Build history of the part. All positions in model axes, mm. Face numbers are marked on the shaded views. A direction names the side the tool comes from. Coordinates: 2 decimals unless noted, no trailing zeros.
from build123d import *
from OCP.BRepFilletAPI import BRepFilletAPI_MakeChamfer

# Parameters (mm, degrees)
SKETCH1_W                       = 194
SKETCH1_H                       = 90
BOSS_EXTRUDE1_DEPTH             = 7
SKETCH3_W                       = 194
SKETCH3_H                       = 90
SKETCH2_W                       = 150
SKETCH2_H                       = 70
CHAMFER1_SIZE                   = 2
SKETCH4_R                       = 2.15
CUT_EXTRUDE1_DEPTH              = 7
SKETCH5_W                       = 150
SKETCH5_H                       = 60
CUT_EXTRUDE2_DEPTH              = 36
SKETCH6_W                       = 150
SKETCH6_H                       = 64
CUT_EXTRUDE3_DEPTH              = 32
SKETCH7_W                       = 6
SKETCH7_H                       = 64
CUT_EXTRUDE4_DEPTH              = 4
SKETCH8_R                       = 2.05
CUT_EXTRUDE5_DEPTH              = 6
CHAMFER2_SIZE                   = 1
CHAMFER2_SIZE2                  = 0.615681714
CHAMFER2_SIZE2_2                = 0.436631997
CHAMFER3_SIZE                   = 0.6
SKIZZE1_W                       = 54.050484576
SKIZZE1_H                       = 12.5
SKIZZE1_W_2                     = 40
SKIZZE1_H_2                     = 21.453027382
AUFSATZ_LINEAR_AUSTRAGEN1_DEPTH = 10
SKIZZE3_W                       = 47.974757712
SKIZZE3_H                       = 1
SCHNITT_LINEAR_AUSTRAGEN2_DEPTH = 4
SKETCH9_W                       = 150
SKETCH9_H                       = 64
CUT_EXTRUDE6_DEPTH              = 32
CHAMFER4_SIZE                   = 0.4


with BuildPart() as part:
    # Sketch1 → Boss-Extrude1 (new body)
    with BuildSketch(Plane(origin=(0, 0, 0), x_dir=(1, 0, 0), z_dir=(0, 1, 0))):
        Rectangle(SKETCH1_W, SKETCH1_H)
    extrude(amount=BOSS_EXTRUDE1_DEPTH)

    # Sketch3 → Loft2 section 0
    with BuildSketch(Plane(origin=(0, 7, 0), x_dir=(1, 0, 0), z_dir=(0, 1, 0))):
        Rectangle(SKETCH3_W, SKETCH3_H)
    # Sketch2 → Loft2 section 1
    with BuildSketch(Plane(origin=(0, 37, 0), x_dir=(1, 0, 0), z_dir=(0, 1, 0))):
        Rectangle(SKETCH2_W, SKETCH2_H)
    loft()

    # Chamfer1
    chamfer1_edges = [part.edges().sort_by_distance(p)[0] for p in [
        (-97, 3.5, 45),
        (97, 3.5, 45),
        (97, 3.5, -45),
        (-97, 3.5, -45),
    ]]
    chamfer(chamfer1_edges, length=CHAMFER1_SIZE)

    # Sketch4 → Cut-Extrude1 (cut)
    with BuildSketch(Plane.XZ):
        with Locations(Location((40, -41.5, 0), (0, 0, 270))):
            Circle(SKETCH4_R)
        with Locations(Location((-40, -41.5, 0), (0, 0, 270))):
            Circle(SKETCH4_R)
    cut_extrude1 = extrude(amount=-CUT_EXTRUDE1_DEPTH, mode=Mode.SUBTRACT)

    # Sketch5 → Cut-Extrude2 (cut)
    with BuildSketch(Plane.XZ):
        Rectangle(SKETCH5_W, SKETCH5_H)
    extrude(amount=-CUT_EXTRUDE2_DEPTH, mode=Mode.SUBTRACT)

    # Mirror1: Cut-Extrude1 across plane
    add(cut_extrude1.mirror(Plane.XY), mode=Mode.SUBTRACT)

    # Sketch6 → Cut-Extrude3 (cut)
    with BuildSketch(Plane.XZ):
        Rectangle(SKETCH6_W, SKETCH6_H)
    extrude(amount=-CUT_EXTRUDE3_DEPTH, mode=Mode.SUBTRACT)

    # Sketch7 → Cut-Extrude4 (cut)
    with BuildSketch(Plane.XZ):
        with Locations((-78, 0)):
            Rectangle(SKETCH7_W, SKETCH7_H)
        with Locations((78, 0)):
            Rectangle(SKETCH7_W, SKETCH7_H)
    extrude(amount=-CUT_EXTRUDE4_DEPTH, mode=Mode.SUBTRACT)

    # Sketch8 → Cut-Extrude5 (cut)
    with BuildSketch(Plane.XZ.offset(-4)):
        with Locations(Location((-78, 25, 0), (0, 0, 270))):
            Circle(SKETCH8_R)
        with Locations(Location((-78, -25, 0), (0, 0, 270))):
            Circle(SKETCH8_R)
        with Locations(Location((78, -25, 0), (0, 0, 90))):
            Circle(SKETCH8_R)
        with Locations(Location((78, 25, 0), (0, 0, 90))):
            Circle(SKETCH8_R)
    extrude(amount=-CUT_EXTRUDE5_DEPTH, mode=Mode.SUBTRACT)

    # Chamfer2: one chamfer whose edges measure the first distance from different faces: ONE call of the kernel's chamfer builder (chamfer() names one face for all edges)
    chamfer2_edges_1 = [part.edges().sort_by_distance(p)[0] for p in [
        (75, 37, 0),
    ]]
    chamfer2_side_1 = [part.faces().sort_by_distance(p)[0] for p in [
        (86.442553469, 21.396517997, 0),
    ]]
    chamfer2_edges_2 = [part.edges().sort_by_distance(p)[0] for p in [
        (0, 37, -35),
    ]]
    chamfer2_side_2 = [part.faces().sort_by_distance(p)[0] for p in [
        (0, 21.370454545, -40.209848485),
    ]]
    chamfer2_edges_3 = [part.edges().sort_by_distance(p)[0] for p in [
        (-75, 37, 0),
    ]]
    chamfer2_side_3 = [part.faces().sort_by_distance(p)[0] for p in [
        (-86.442553469, 21.396517997, 0),
    ]]
    chamfer2_edges_4 = [part.edges().sort_by_distance(p)[0] for p in [
        (0, 37, 35),
    ]]
    chamfer2_side_4 = [part.faces().sort_by_distance(p)[0] for p in [
        (0, 21.370454545, 40.209848485),
    ]]
    chamfer2 = BRepFilletAPI_MakeChamfer(part.part.solid().wrapped)
    for e in chamfer2_edges_1:
        chamfer2.Add(CHAMFER2_SIZE, CHAMFER2_SIZE2, e.wrapped, chamfer2_side_1[0].wrapped)  # the first distance lies on this face
    for e in chamfer2_edges_2:
        chamfer2.Add(CHAMFER2_SIZE, CHAMFER2_SIZE2_2, e.wrapped, chamfer2_side_2[0].wrapped)  # the first distance lies on this face
    for e in chamfer2_edges_3:
        chamfer2.Add(CHAMFER2_SIZE, CHAMFER2_SIZE2, e.wrapped, chamfer2_side_3[0].wrapped)  # the first distance lies on this face
    for e in chamfer2_edges_4:
        chamfer2.Add(CHAMFER2_SIZE, CHAMFER2_SIZE2_2, e.wrapped, chamfer2_side_4[0].wrapped)  # the first distance lies on this face
    add(Compound.cast(chamfer2.Shape()), mode=Mode.REPLACE)

    # Chamfer3
    chamfer3_edges = [part.edges().sort_by_distance(p)[0] for p in [
        (0, 0, 45),
        (97, 0, 0),
        (-97, 0, 0),
        (0, 0, -45),
        (-96, 0, -44),
        (96, 0, -44),
        (96, 0, 44),
        (-96, 0, 44),
    ]]
    chamfer(chamfer3_edges, length=CHAMFER3_SIZE)

    # Skizze1 → Aufsatz-Linear austragen1 (add)
    with BuildSketch(Plane.XZ.offset(-36)):
        with Locations((0, -23.75)):
            Rectangle(SKIZZE1_W, SKIZZE1_H)
        with Locations((0, 23.75)):
            Rectangle(SKIZZE1_W, SKIZZE1_H)
        with Locations((55, 0)):
            Rectangle(SKIZZE1_W_2, SKIZZE1_H_2)
    extrude(amount=AUFSATZ_LINEAR_AUSTRAGEN1_DEPTH)

    # Skizze3 → Schnitt-Linear austragen2 (cut)
    with BuildSketch(Plane(origin=(0, 36, 0), x_dir=(-1, 0, 0), z_dir=(0, -1, 0))):
        with Locations((51.012621144, -30.5)):
            Rectangle(SKIZZE3_W, SKIZZE3_H)
        with Locations((-51.012621144, -30.5)):
            Rectangle(SKIZZE3_W, SKIZZE3_H)
        with Locations((51.012621144, 30.5)):
            Rectangle(SKIZZE3_W, SKIZZE3_H)
        with Locations((-51.012621144, 30.5)):
            Rectangle(SKIZZE3_W, SKIZZE3_H)
    extrude(amount=SCHNITT_LINEAR_AUSTRAGEN2_DEPTH, mode=Mode.SUBTRACT)

    # Sketch9 → Cut-Extrude6 (cut)
    with BuildSketch(Plane.XZ.offset(-4)):
        Rectangle(SKETCH9_W, SKETCH9_H)
    extrude(amount=-CUT_EXTRUDE6_DEPTH, mode=Mode.SUBTRACT)

    # Chamfer4
    chamfer4_edges = [part.edges().sort_by_distance(p)[0] for p in [
        (40, 0, -39.35),
        (-40, 0, -39.35),
        (40, 0, 39.35),
        (-40, 0, 39.35),
    ]]
    chamfer(chamfer4_edges, length=CHAMFER4_SIZE)


solid = part.part
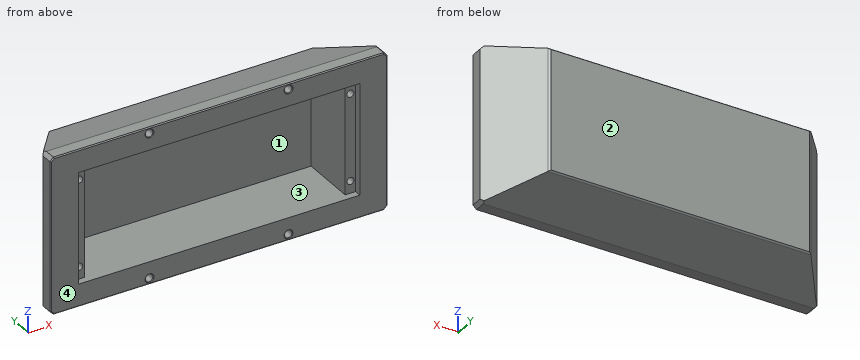
(1) Two-plate mould, pull along Z, no slides. Class the marked faces 1 and 2: pulls with the +Z half, pulls with the -Z half, needs draft (parallel to the pull), parting line crosses it, or undercut.
(2) Probe L1, parallel to Z at x = 78, y = 6; L2, parallel to X at y = 2, z = -41.5; L3, parallel to X at y = 2.5, z = -27. List the from-to ranges inside material, lowest first.
(3) Flat gauge pins, fed straight in: P1, Ø6.5, axis at x = 78, z = 25, coming from the +Y side; P2, Ø1.5, axis at x = 22, y = 21.5, coming from the +Z side; P3, Ø4.5, axis at x = 78.5, z = -24.5, coming from the -Y side. Where does each tip first touch, or does it go through?
(4) 3-axis set-ups, long thin cutter, end or side, ignore diameter. For the marked faces 3 and 4: which of +Z, -Z, +X, -X, +Y, -Y reach the whole face in a straight line?
Results:
1. face 1: undercut
1. face 2: needs draft
2. L1: z = -45 to -27.05, -22.95 to 22.95, 27.05 to 45
2. L2: x = -97 to -42.15, -37.85 to 37.85, 42.15 to 97
2. L3: x = -97 to -81, 81 to 97
3. P1: stops at y = 36.76
3. P2: stops at z = 40.42
3. P3: stops at y = 4
4. face 3: -Y
4. face 4: +Z, -Z, +X, -X, -Y
